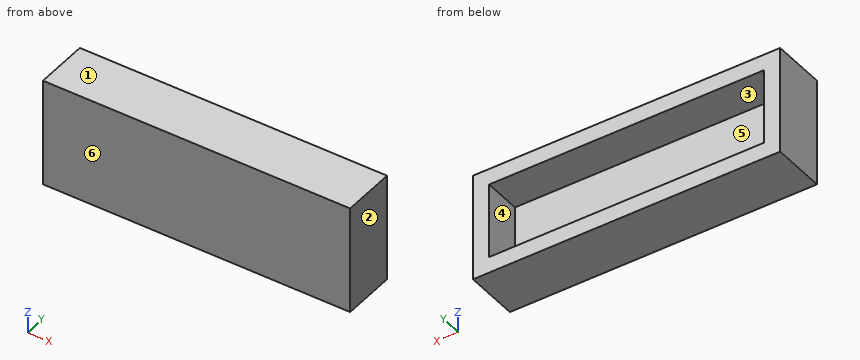
Autodesk Inventor part; units mm, degrees
ref_plane "YZ Plane" through (0, 0, 0) normal (1, 0, 0) x (0, 1, 0)
ref_plane "XZ Plane" through (0, 0, 0) normal (0, 1, 0) x (-1, 0, 0)
ref_plane "XY Plane" through (0, 0, 0) normal (0, 0, 1) x (1, 0, 0)
sketch "スケッチ1" plane through (0, 0, 0) normal (0, 1, 0) x (-1, 0, 0)
  line L0 (0, 0) -> (57, 0)
  line L1 (57, 0) -> (57, -20)
  line L2 (57, -20) -> (0, -20)
  line L3 (0, -20) -> (0, 0)
  dimension "d0" = 20
  dimension "d1" = 57
extrude "押し出し1" add sketch "スケッチ1" along normal blind 10
shell "シェル2" thickness 3 removed faces 1 at (-19, 10, -6.6667)
properties part number "suply_hub"
Model file for the job. Use its own axes, mm. Face numbers are marked on the shaded views. A direction names the side the tool comes from. Give positions to 0.01 mm unless a question says otherwise; leave off trailing zeros. Loops run counter-clockwise (first coordinate to the right, second up) from the corner with the lowest first, then second, coordinate; pieces in that order, holes last. Notation, with made-up numbers: (0, 19) -> (32, 19) arc R32 cw to (32, 54) -> close; hole circle Ø9 at (63.25, 84.25). An arc over 180 degrees is marked (long way). Use a Markdown table: item, result. Add a question column.
(1) Tool access for the marked faces 5 and 6: list every direction of +Z, -Z, +X, -X, +Y, -Y with a clear straight run to the whole face (end or side of a thin tool).
(2) Slice it at C-C on z = -15. List the corners of the cut face in (x, y), and give its area (3 significant figures).
(3) Mould opens along Z. For the marked faces 1, 2, 3 and 4 say: +Z half, -Z half, draft (parallel to the pull), parting line (faces both ways), or undercut.
(4) Wall check: line 1 along X through (y, z) = (7, -10); line 2 along Z through (x, y) = (-35, 5.75); line 3 along Y through (x, z) = (-53, -3.5). Give the ranges that are in metal, low to high.
(5) Drop a flat-ended pin along its axis: pin 1 Ø10 at (x, z) = (-25, -12.5) entering from -Y. Give the stop position or say it passes through.
(6) Slice it at B-B on y = 7.25. List the corners of the cut face in (x, z).
(7) Slice it at A-A on x = -24. List the corners of the cut face in (y, z).
Filled sheet:
| question | item | result |
|---|---|---|
| 1 | face 5 | +Y |
| 1 | face 6 | +Z, -Z, +X, -X, -Y |
| 2 | outline | (-57, 0) -> (0, 0) -> (0, 10) -> (-3, 10) -> (-3, 3) -> (-54, 3) -> (-54, 10) -> (-57, 10) -> close |
| 2 | area | 213 mm2 |
| 3 | face 1 | +Z half |
| 3 | face 2 | draft |
| 3 | face 3 | undercut |
| 3 | face 4 | undercut |
| 4 | line 1 | -57 to -54, -3 to 0 |
| 4 | line 2 | -20 to -17, -3 to 0 |
| 4 | line 3 | 0 to 3 |
| 5 | pin 1 | y = 0 |
| 6 | outline | (-57, -20) -> (0, -20) -> (0, 0) -> (-57, 0) -> close; hole (-54, -17) -> (-3, -17) -> (-3, -3) -> (-54, -3) -> close |
| 7 | outline | (0, -20) -> (10, -20) -> (10, -17) -> (3, -17) -> (3, -3) -> (10, -3) -> (10, 0) -> (0, 0) -> close |
